from build123d import *

# Parameters (mm, degrees)
EXTRUDE_1_DEPTH     = 2.5
SKETCH_2_R          = 1
CUT_EXTRUDE_1_DEPTH = 28.041634566


with BuildPart() as part:
    # 草图1 → 凸台-拉伸1 (new, symmetric)
    with BuildSketch(Plane.XY):
        Polygon((0, 0), (13, 0), (13, -7), (11, -7), (11, -2), (0, -2), align=None)
    extrude_1 = extrude(amount=EXTRUDE_1_DEPTH, both=True)

    # 镜向1: 凸台-拉伸1 across plane
    add(extrude_1.mirror(Plane(origin=(0, 0, 0), x_dir=(0, 0, 1), z_dir=(1, 0, 0))))

    # 草图2 → 切除-拉伸1 (cut, through all)
    with BuildSketch(Plane(origin=(13, 0, 0), x_dir=(0, 0, -1), z_dir=(1, 0, 0))):
        with Locations((0, -4.5)):
            Circle(SKETCH_2_R)
    extrude(amount=-CUT_EXTRUDE_1_DEPTH, mode=Mode.SUBTRACT)

    # 草图3 → 旋转1 (revolve)
    with BuildSketch(Plane(origin=(8, 0, 0), x_dir=(0, 0, -1), z_dir=(1, 0, 0))):
        with BuildLine():
            Line((0, 0), (0, 4.5))
            ThreePointArc((0, 4.5), (1.915810353, 3.074169567), (1.1, 0.829670691))
            Line((1.1, 0.829670691), (1.1, 0))
            Line((1.1, 0), (0, 0))
        make_face()
    revolve(axis=Axis((8, 0, 0), (0, 1, 0)))

    # 草图4 → 旋转2 (revolve)
    with BuildSketch(Plane.ZY.offset(8), mode=Mode.PRIVATE) as revolve_2_sk:
        with BuildLine():
            Line((0, 0), (0, 4.5))
            ThreePointArc((0, 4.5), (1.915810353, 3.074169567), (1.1, 0.829670691))
            Line((1.1, 0.829670691), (1.1, 0))
            Line((1.1, 0), (0, 0))
        make_face()
    revolve(revolve_2_sk.sketch.rotate(Axis((-8, 0, 0), (0, 1, 0)), 180), axis=Axis((-8, 0, 0), (0, 1, 0)))


solid = part.part
Could you check a few things on this model? Use its own coordinates, in mm. A direction names the side the tool comes from. Give positions to 0.01 mm unless a question says otherwise; leave off trailing zeros. Write each loop counter-clockwise with the first axis right and the second up, starting at its lowest first coordinate (ties: lowest second). Pieces come first, ordered by that corner, then holes. Notation, with made-up numbers: (21, 61.5) - (26, 61.5) arc R18 ccw to (26, 92.5) - close; hole circle Ø11 at (-31.75, -26.75). An arc over 180 degrees is marked (long way). Use CSV: the item, a comma, the result in double quotes. Start each with the question number.
Item 1: I'm going to push flat-ended pins straight in: pin 1 (3 mm diameter, centred on x = 5, z = -0.5, fed in from +Y); pin 2 (3 mm diameter, centred on y = -4.5, z = 0, fed in from -X). Where does each tip first touch, or does it pass through?
Item 2: I want a section at D-D, the plane x = 9.5. Please give me the cut outline in (y, z).
Item 3: I want a section at A-A, the plane y = -4.5. Please give me the cut outline in (x, z), then the cut area to 3 significant figures.
Item 4: If we mould it in two halves opening along X, with no side actions, what happens to faces 1 (the face through (-11.99, -3.51, 0.13)), 2 (the face through (-13, -3, 0)), 3 (the face through (-11, -6, 0)), 4 (the face through (-6.926, 0.409, 0.238))? For each: pulls with the +X half, pulls with the -X half, needs draft (parallel to the pull), parting line crosses it, or undercut.
Item 5: I want a section at B-B, the plane z = 0. Please give me the cut outline in (x, y), then the cut area to 3 significant figures.
Item 6: I want a section at C-C, the plane x = -8. Please give me the cut outline in (y, z).
Item 7: If I drill on line 1 along X through (y, z) = (-5, -2); line 2 along Y through (x, z) = (-12.5, 0); line 3 along Y through (x, z) = (10.5, 1.7), over which ranges is the centre line in solid material (lowest first)?
Item 8: For faces 5 (the face through (9.074, 0.409, 0.238)), 6 (the face through (12, -7, 0)), 7 (the face through (11, -6, 0)), which set-ups out of +Z, -Z, +X, -X, +Y, -Y let a thin tool reach every point of the face, with its end or its side?
Findings:
1,pin 1,"stops at y = 3.77"
1,pin 2,"stops at x = -13"
2,outline,"(-2, -2.5) - (0, -2.5) - (0, 2.5) - (-2, 2.5) - close; circle Ø2.65 at (2.5, 0)"
3,outline,"(-13, -2.5) - (-11, -2.5) - (-11, -1) - (-13, -1) - close; (-13, 1) - (-11, 1) - (-11, 2.5) - (-13, 2.5) - close; (11, -2.5) - (13, -2.5) - (13, -1) - (11, -1) - close; (11, 1) - (13, 1) - (13, 2.5) - (11, 2.5) - close"
3,area,"12.0 mm2"
4,face 1,"needs draft"
4,face 2,"pulls with the -X half"
4,face 3,"undercut"
4,face 4,"undercut"
5,outline,"(-13, -7) - (-11, -7) - (-11, -5.5) - (-13, -5.5) - close; (-13, -3.5) - (-11, -3.5) - (-11, -2) - (11, -2) - (11, -3.5) - (13, -3.5) - (13, 0) - (9.1, 0) - (9.1, 0.83) arc R2 ccw (long way) to (6.9, 0.83) - (6.9, 0) - (-6.9, 0) - (-6.9, 0.83) arc R2 ccw (long way) to (-9.1, 0.83) - (-9.1, 0) - (-13, 0) - close; (11, -7) - (13, -7) - (13, -5.5) - (11, -5.5) - close"
5,area,"91.8 mm2"
6,outline,"(-2, -2.5) - (0, -2.5) - (0, -1.1) - (0.83, -1.1) arc R2 ccw (long way) to (0.83, 1.1) - (0, 1.1) - (0, 2.5) - (-2, 2.5) - close"
7,line 1,"x = -13 to -11, 11 to 13"
7,line 2,"y = -7 to -5.5, -3.5 to 0"
7,line 3,"y = -2 to 0"
8,face 5,"none"
8,face 6,"+Z, -Z, +X, -X, -Y"
8,face 7,"+Z, -Z, -Y"
